Work out the finished part from the listing and answer in its coordinate system (mm). A direction names the side the tool comes from. Coordinates: 2 decimals unless noted, no trailing zeros. Order: outer loops, then holes, each group sorted by start corner. A loop starts at its lowest first (then second) coordinate and runs counter-clockwise, first axis right, second up. Notation, with made-up numbers: M 73,-17.5 L 96,-17.5 A19 ccw 96,6.5 Z; hole C -9,68.5 d2. An arc over 180 degrees is marked long. Use a Markdown table: item, result. Add a question column.
from build123d import *

# Parameters (mm, degrees)
SKETCH1_W           = 12
SKETCH1_H           = 8
BOSS_EXTRUDE1_DEPTH = 2
SKETCH2_W           = 12
SKETCH2_H           = 3.7
BOSS_EXTRUDE2_DEPTH = 2.5
CUT_EXTRUDE1_DEPTH  = 15.088026831


with BuildPart() as part:
    # Sketch1 → Boss-Extrude1 (new body)
    with BuildSketch(Plane(origin=(0, 0, 0), x_dir=(1, 0, 0), z_dir=(0, 1, 0))):
        with Locations((6, 0)):
            Rectangle(SKETCH1_W, SKETCH1_H)
    extrude(amount=BOSS_EXTRUDE1_DEPTH)

    # Sketch2 → Boss-Extrude2 (add)
    with BuildSketch(Plane(origin=(0, 2, 0), x_dir=(1, 0, 0), z_dir=(0, 1, 0))):
        with Locations((6, 0)):
            Rectangle(SKETCH2_W, SKETCH2_H)
    extrude(amount=BOSS_EXTRUDE2_DEPTH)

    # Sketch3 → Cut-Extrude1 (cut, through all)
    with BuildSketch(Plane.XY.offset(1.85)):
        with BuildLine():
            Line((4.5, 3.5), (4.5, 5))
            Line((4.5, 5), (7.5, 5))
            Line((7.5, 5), (7.5, 3.5))
            ThreePointArc((7.5, 3.5), (6, 2), (4.5, 3.5))
        make_face()
    extrude(amount=-CUT_EXTRUDE1_DEPTH, mode=Mode.SUBTRACT)


solid = part.part
(1) A cutting plane is placed at C-C on x = 8.75. Write down the section's boundary in (y, z), plus the area to 4 significant figures.
(2) The mould has two halves that part along X. Classify faces 4 (the cylindrical face through (6, 2, 0)), 5 (the flat face through (0, 2, 0)), 6 (the flat face through (6, 0, 0)): pulls with the +X half, pulls with the -X half, needs draft (parallel to the pull), parting line crosses it, or undercut.
(3) Straight lines are drawn through the part: line 1 (Y direction, x = 3.75, z = -3); line 2 (X direction, y = 2.65, z = 1.75); line 3 (Z direction, x = 1.5, y = 3.85). For each, find the intervals that lie inside material, in ascending order.
(4) Which of the six approach directions +Z, -Z, +X, -X, +Y, -Y give full straight-line access (tool end or side, diameter ignored) to faces 1 (the flat face through (6, 2, 3)), 2 (the flat face through (4.5, 4, 0)), 3 (the flat face through (10, 3, -1.85))?
(5) A cutting plane is placed at A-A on y = 3.65. Write down the section's boundary in (x, z).
(6) A cutting plane is placed at D-D on z = 2. Write down the section's boundary in (x, y).
(7) A cutting plane is placed at B-B on z = -0.5. Write down the section's boundary in (x, y), plus the area to 3 significant figures.
(8) Given P1, Ø1.1, axis at x = 6, z = -3.5, coming from the +Y side; P2, Ø4, axis at x = 3, z = -2.5, coming from the +Y side; P3, Ø2, axis at x = 10, y = 3.5, coming from the -Z side; P4, Ø0.8, axis at x = 3, y = 3.5, coming from the +Z side, each flat-ended and moving along its own axis, determine where each tip first touches the part or whether it passes through.
From the geometry:
| question | item | result |
|---|---|---|
| 1 | outline | M 0,-4 L 2,-4 L 2,-1.85 L 4.5,-1.85 L 4.5,1.85 L 2,1.85 L 2,4 L 0,4 Z |
| 1 | area | 25.25 mm2 |
| 2 | face 4 | undercut |
| 2 | face 5 | pulls with the -X half |
| 2 | face 6 | needs draft |
| 3 | line 1 | y = 0 to 2 |
| 3 | line 2 | x = 0 to 4.76, 7.24 to 12 |
| 3 | line 3 | z = -1.85 to 1.85 |
| 4 | face 1 | +Z, +X, -X, +Y |
| 4 | face 2 | +Z, -Z, +Y |
| 4 | face 3 | -Z, +X, -X, +Y |
| 5 | outline | M 0,-1.85 L 4.5,-1.85 L 4.5,1.85 L 0,1.85 Z; M 7.5,-1.85 L 12,-1.85 L 12,1.85 L 7.5,1.85 Z |
| 6 | outline | M 0,0 L 12,0 L 12,2 L 0,2 Z |
| 7 | outline | M 0,0 L 12,0 L 12,4.5 L 7.5,4.5 L 7.5,3.5 A1.5 cw 4.5,3.5 L 4.5,4.5 L 0,4.5 Z |
| 7 | area | 47.5 mm2 |
| 8 | P1 | stops at y = 2 |
| 8 | P2 | stops at y = 4.5 |
| 8 | P3 | stops at z = -1.85 |
| 8 | P4 | stops at z = 1.85 |
